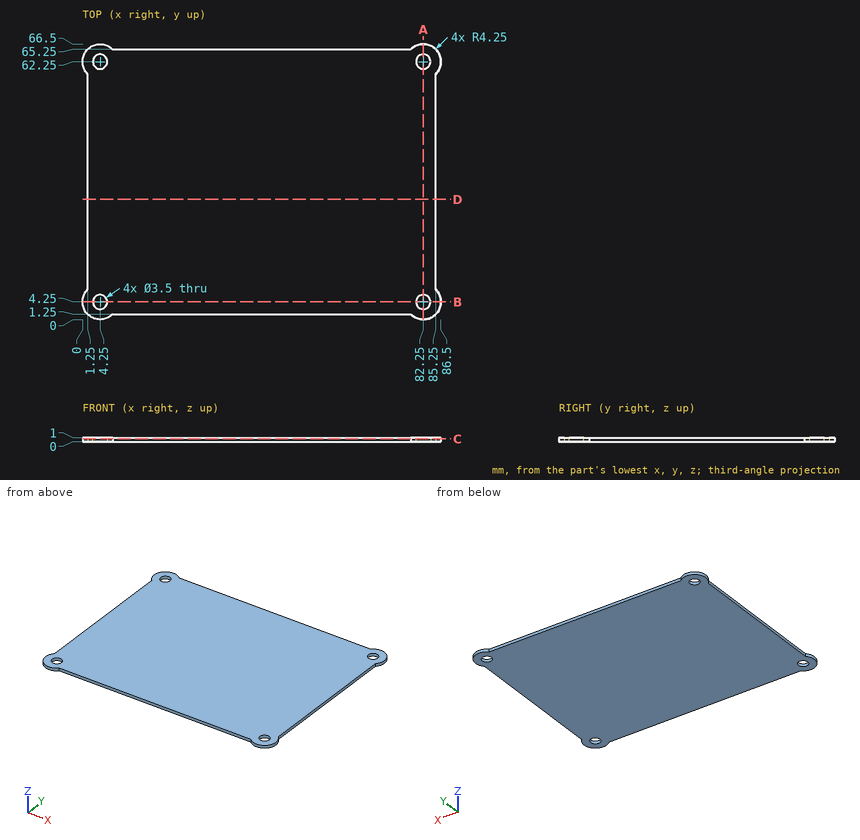
Can you work these out from the drawing? Everything is in mm from the part's minimum corner. Give positions to 0.01 mm unless a question says otherwise; leave off trailing zeros. Order: outer loops, then holes, each group sorted by start corner. A loop starts at its lowest first (then second) coordinate and runs counter-clockwise, first axis right, second up. Notation, with made-up numbers: M -17.5,3.5 L 17.5,3.5 A16 cw 17.5,18.5 Z; hole C 45,76.5 d8. An arc over 180 degrees is marked long. Use a Markdown table: item, result. Add a question column.
Item 1: Will this pin go through, and if not, where does the flat tip stop? pin 1 (3 mm diameter, centred on x = 82.25, y = 62.25, fed in from -Z).
Item 2: Suppose I cut it at B-B (y = 4.25). List the corners of the cut face in (x, z) for me, then the cut area to 3 significant figures.
Item 3: Suppose I cut it at C-C (z = 0.7). List the corners of the cut face in (x, y) for me, then the cut area to 3 significant figures.
Item 4: Suppose I cut it at A-A (x = 82.25). List the corners of the cut face in (y, z) for me.
Item 5: If I drill on L1, parallel to Y at x = 82.5, z = 0.6; L2, parallel to X at y = 4.5, z = 0.4; L3, parallel to Y at x = 42.5, z = 0.75, over which ranges is the centre line in solid material (lowest first)? Write a range as [from, to].
Item 6: Suppose I cut it at D-D (y = 29). List the corners of the cut face in (x, z) for me.
Answer sheet:
| question | item | result |
|---|---|---|
| 1 | pin 1 | passes through |
| 2 | outline | M 0,0 L 2.5,0 L 2.5,1 L 0,1 Z; M 6,0 L 80.5,0 L 80.5,1 L 6,1 Z; M 84,0 L 86.5,0 L 86.5,1 L 84,1 Z |
| 2 | area | 79.5 mm² |
| 3 | outline | M 1.25,7.26 A4.25 ccw 7.26,1.25 L 79.24,1.25 A4.25 ccw 85.25,7.26 L 85.25,59.24 A4.25 ccw 79.24,65.25 L 7.26,65.25 A4.25 ccw 1.25,59.24 Z; hole C 4.25,4.25 d3.5; hole C 4.25,62.25 d3.5; hole C 82.25,4.25 d3.5; hole C 82.25,62.25 d3.5 |
| 3 | area | 5,380 mm² |
| 4 | outline | M 0,0 L 2.5,0 L 2.5,1 L 0,1 Z; M 6,0 L 60.5,0 L 60.5,1 L 6,1 Z; M 64,0 L 66.5,0 L 66.5,1 L 64,1 Z |
| 5 | L1 | y = [0.01, 2.52], [5.98, 60.52], [63.98, 66.49] |
| 5 | L2 | x = [0.01, 2.52], [5.98, 80.52], [83.98, 86.49] |
| 5 | L3 | y = [1.25, 65.25] |
| 6 | outline | M 1.25,0 L 85.25,0 L 85.25,1 L 1.25,1 Z |
